Can you work these out from the drawing? Everything is in mm from the part's minimum corner. A direction names the side the tool comes from. Coordinates: 2 decimals unless noted, no trailing zeros. Order: outer loops, then holes, each group sorted by start corner. A loop starts at its lowest first (then second) coordinate and runs counter-clockwise, first axis right, second up. Notation, with made-up numbers: (25.25, 51) - (54.25, 51) arc R17 cw to (54.25, 63) - close; hole circle Ø1 at (83.25, -7). An arc over 180 degrees is marked (long way). Answer as CSV lines item,"result". Start each with the question number.
Item 1: I need wall thicknesses on line 1 (Y direction, x = 12.5, z = 1.7); line 2 (X direction, y = 5.75, z = 3.5); line 3 (Y direction, x = 20.75, z = 4). Which ranges of each line are inside material? Lowest first, please.
Item 2: On a 3-axis mill with a long thin cutter (end or side, diameter ignored), from which of +Z, -Z, +X, -X, +Y, -Y can I reach the whole of each face in a straight line? I mean the marked faces 4, 5, 6 and 7. Say none if no direction works.
Item 3: Imagine slicing it at D-D on x = 12.5. List the corners of the cut face in (y, z) for me.
Item 4: We'd pull the mould along Y, two halves only. Please class the marked faces 1, 2 and 3: pulls with the +Y half, pulls with the -Y half, needs draft (parallel to the pull), parting line crosses it, or undercut.
Item 5: Imagine slicing it at A-A on z = 2.5. List the corners of the cut face in (x, y) for me.
Item 6: Imagine slicing it at B-B on x = 2.75. List the corners of the cut face in (y, z) for me, and give its area (3 significant figures).
Item 7: Imagine slicing it at C-C on y = 21.75. List the corners of the cut face in (x, z) for me, and give its area (3 significant figures).
Item 8: I'm going to push flat-ended pins straight in: pin 1 (2.5 mm diameter, centred on y = 14.5, z = 4, fed in from -X); pin 2 (1.9 mm diameter, centred on x = 2.5, y = 27.5, fed in from -Z); pin 3 (13.5 mm diameter, centred on x = 13.5, y = 14, fed in from +Z). Where does each tip first touch, or does it pass through?
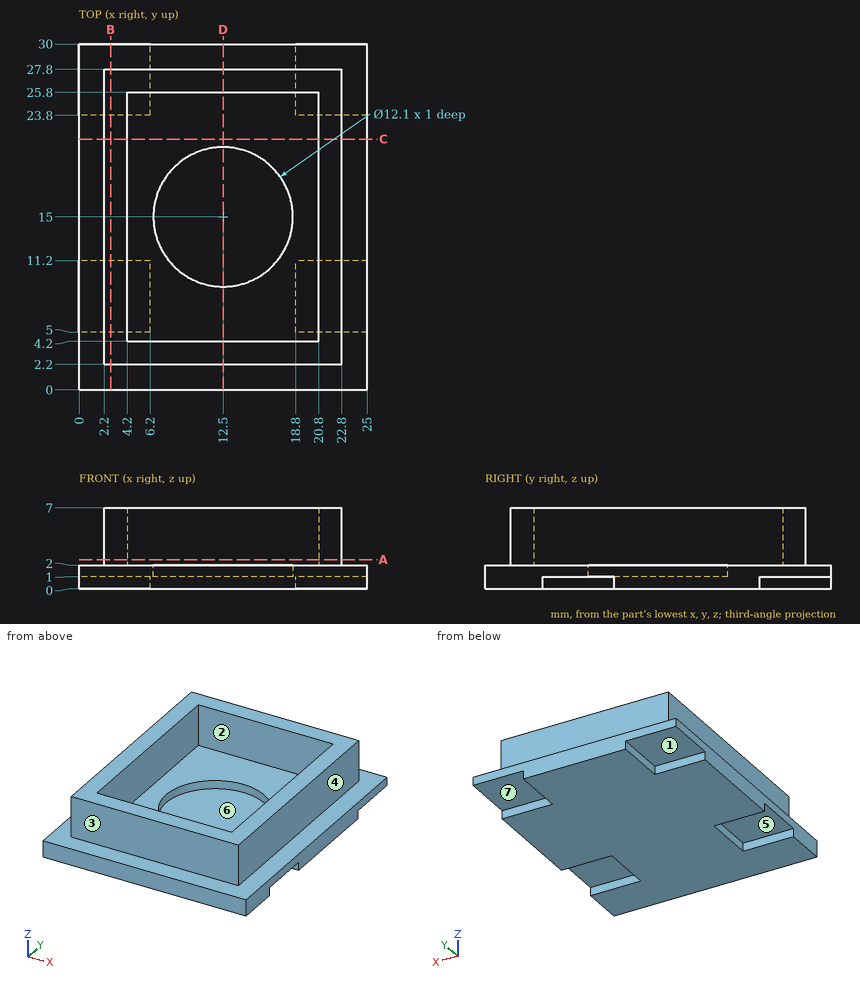
Responses:
1,line 1,"y = 0 to 8.95, 21.05 to 30"
1,line 2,"x = 2.2 to 4.2, 20.8 to 22.8"
1,line 3,"y = 2.2 to 4.2, 25.8 to 27.8"
2,face 4,"+Z, +X, +Y, -Y"
2,face 5,"-Z, -X"
2,face 6,"+Z"
2,face 7,"-Z, +X, +Y"
3,outline,"(0, 0) - (30, 0) - (30, 2) - (27.8, 2) - (27.8, 7) - (25.8, 7) - (25.8, 2) - (21.05, 2) - (21.05, 1) - (8.95, 1) - (8.95, 2) - (4.2, 2) - (4.2, 7) - (2.2, 7) - (2.2, 2) - (0, 2) - close"
4,face 1,"needs draft"
4,face 2,"undercut"
4,face 3,"pulls with the -Y half"
5,outline,"(2.2, 2.2) - (22.8, 2.2) - (22.8, 27.8) - (2.2, 27.8) - close; hole (4.2, 4.2) - (20.8, 4.2) - (20.8, 25.8) - (4.2, 25.8) - close"
6,outline,"(0, 0) - (5, 0) - (5, 1) - (11.2, 1) - (11.2, 0) - (23.8, 0) - (23.8, 1) - (30, 1) - (30, 2) - (27.8, 2) - (27.8, 7) - (2.2, 7) - (2.2, 2) - (0, 2) - close"
6,area,"176 mm^2"
7,outline,"(0, 0) - (25, 0) - (25, 2) - (22.8, 2) - (22.8, 7) - (20.8, 7) - (20.8, 2) - (4.2, 2) - (4.2, 7) - (2.2, 7) - (2.2, 2) - (0, 2) - close"
7,area,"70.0 mm^2"
8,pin 1,"stops at x = 2.2"
8,pin 2,"stops at z = 1"
8,pin 3,"stops at z = 2"
